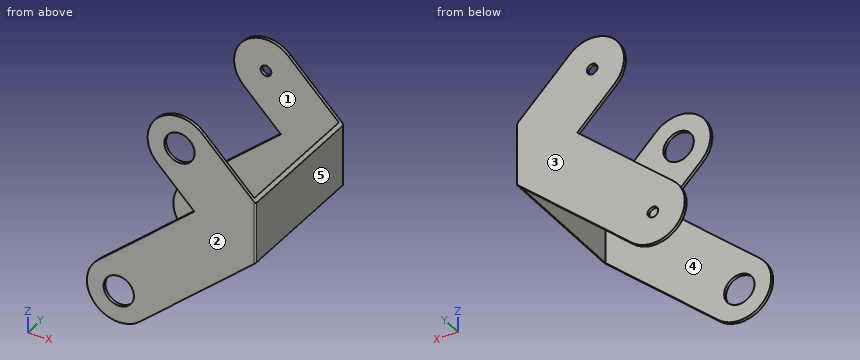
```python
from build123d import *

# Parameters (mm, degrees)
EXTRUDE_1_DEPTH             = 47
SHELL_1_T                   = -1
FILLET_2_R                  = 0.5
HOLE_WIZARD_3_5_3_5_1_D     = 3.5
HOLE_WIZARD_3_5_3_5_1_DEPTH = 1
HOLE_WIZARD_10_0_10_3_D     = 10
HOLE_WIZARD_10_0_10_3_DEPTH = 1


with BuildPart() as part:
    # 草图1 → 凸台-拉伸1 (new body)
    with BuildSketch(Plane(origin=(0, 0, 0), x_dir=(1, 0, 0), z_dir=(0, 1, 0))):
        with BuildLine():
            Line((25, 30), (-13.135780284, 62.94559549))
            ThreePointArc((-13.135780284, 62.94559549), (-27.94559549, 61.864219716), (-26.864219716, 47.05440451))
            Line((-26.864219716, 47.05440451), (4.883538541, 19.627437146))
            Line((4.883538541, 19.627437146), (-7.392601402, 7.456503505))
            ThreePointArc((-7.392601402, 7.456503505), (-7.456503505, -7.392601402), (7.392601402, -7.456503505))
            Line((7.392601402, -7.456503505), (25, 10))
            Line((25, 10), (25, 30))
        make_face()
    extrude(amount=EXTRUDE_1_DEPTH)

    # 抽壳1
    shell_1_openings = [part.faces().sort_by_distance(p)[0] for p in [
        (5.932109858, 23.5, -46.472797745),
        (16.196300701, 23.5, -1.271748248),
        (-7.456503505, 23.5, 7.392601402),
        (-1.25453143, 23.5, -13.541970325),
        (-10.990340588, 23.5, -33.340920828),
        (-27.94559549, 23.5, -61.864219716),
    ]]
    offset(amount=SHELL_1_T, openings=shell_1_openings, kind=Kind.INTERSECTION)

    # 圆角2
    fillet_2_edges = [part.edges().sort_by_distance(p)[0] for p in [
        (25, 47, -20),
        (25, 0, -20),
    ]]
    fillet(fillet_2_edges, radius=FILLET_2_R)

    # Ø3.5 (3.5) 直径槽口1
    with Locations(Plane(origin=(0, 47, 0), x_dir=(1, 0, 0), z_dir=(0, 1, 0))):
        with Locations((0, 0), (-20, 55)):
            Hole(HOLE_WIZARD_3_5_3_5_1_D / 2, depth=HOLE_WIZARD_3_5_3_5_1_DEPTH)

    # Ø10.0 (10) 直径槽口3
    with Locations(Plane(origin=(0, 0, 0), x_dir=(-1, 0, 0), z_dir=(0, -1, 0))):
        with Locations((0, 0), (20, 55)):
            Hole(HOLE_WIZARD_10_0_10_3_D / 2, depth=HOLE_WIZARD_10_0_10_3_DEPTH)


solid = part.part
```
Work out the finished part from the listing and answer in its coordinate system (mm). Face numbers are marked on the shaded views. A direction names the side the tool comes from. Coordinates: 2 decimals unless noted, no trailing zeros. Loops run counter-clockwise (first coordinate to the right, second up) from the corner with the lowest first, then second, coordinate; pieces in that order, holes last. Notation, with made-up numbers: M 8.5,76.5 L 64.5,76.5 A20 cw 64.5,93.5 Z; hole C 78.25,58 d10. An arc over 180 degrees is marked long. Use CSV: the item, a comma, the result in double quotes. Start each with the question number.
(1) Find section A-A, the plane z = -48.5. Give the vertices of the cut face in (x, y), then the cut area to 3 significant figures.
(2) For a pull along Y with two mould halves and no side action, classify the marked faces 3, 4 and 5 as +Y half, -Y half, draft (parallel to the pull), parting line (faces both ways), or undercut.
(3) Find section B-B, the plane x = 0. Give the vertices of the cut face in (y, z), then the cut area to 3 significant figures.
(4) Find section C-C, the plane x = 19.5. Give the vertices of the cut face in (y, z).
(5) Find section D-D, the plane x = -8.5. Give the vertices of the cut face in (y, z).
(6) Consider line 1 (Y direction, x = 2, z = -39); line 2 (Z direction, x = 0, y = 0.45); line 3 (X direction, y = 19, z = -26). Determine where each line is inside the solid, lowest interval first.
(7) For the marked faces 1 and 2, determine the directions among +Z, -Z, +X, -X, +Y, -Y from which every point of the face is accessible in a straight line to the end or side of a thin tool.
(8) Given pin 1 Ø6 at (y, z) = (30, -18.5) entering from -X, flat-ended and moving along its own axis, determine where the tip first touches the part or whether it passes through.
Recorded:
1,outline,"M -28.25,0 L 3.59,0 L 3.59,1 L -28.25,1 Z; M -28.25,46 L 3.59,46 L 3.59,47 L -28.25,47 Z"
1,area,"63.7 mm^2"
2,face 3,"+Y half"
2,face 4,"undercut"
2,face 5,"draft"
3,outline,"M 0,-51.6 L 1,-51.6 L 1,-23.85 L 0,-23.85 Z; M 0,-14.79 L 1,-14.79 L 1,-5 L 0,-5 Z; M 0,5 L 1,5 L 1,10.5 L 0,10.5 Z; M 46,-51.6 L 47,-51.6 L 47,-23.85 L 46,-23.85 Z; M 46,-14.79 L 47,-14.79 L 47,-1.75 L 46,-1.75 Z; M 46,1.75 L 47,1.75 L 47,10.5 L 46,10.5 Z"
3,area,"92.6 mm^2"
4,outline,"M 0,-34.75 L 1,-34.75 L 1,-4.55 L 0,-4.55 Z; M 46,-34.75 L 47,-34.75 L 47,-4.55 L 46,-4.55 Z"
5,outline,"M 0,-58.94 L 1,-58.94 L 1,-31.19 L 0,-31.19 Z; M 0,-6.16 L 1,-6.16 L 1,6.16 L 0,6.16 Z; M 46,-58.94 L 47,-58.94 L 47,-31.19 L 46,-31.19 Z; M 46,-6.16 L 47,-6.16 L 47,6.16 L 46,6.16 Z"
6,line 1,"y = 0 to 1, 46 to 47"
6,line 2,"z = -51.6 to -23.85, -14.79 to -5, 5 to 10.5"
6,line 3,"x = 24 to 25"
7,face 1,"+Z, -Z, -X"
7,face 2,"+Z, -Z, +X, -X, -Y"
8,pin 1,"stops at x = 24"
